Autodesk Inventor part; units mm, degrees
ref_plane "YZ Plane" through (0, 0, 0) normal (1, 0, 0) x (0, 1, 0)
ref_plane "XZ Plane" through (0, 0, 0) normal (0, 1, 0) x (-1, 0, 0)
ref_plane "XY Plane" through (0, 0, 0) normal (0, 0, 1) x (1, 0, 0)
sketch "Sketch1" plane through (0, 0, 0) normal (0, 1, 0) x (-1, 0, 0)
  line L0 (0, 0) -> (170, 0)
  line L1 (170, 0) -> (170, 10)
  line L2 (170, 10) -> (0, 10)
  line L3 (0, 10) -> (0, 0)
  dimension "d0" = 170
  dimension "d1" = 10
extrude "Extrusion1" add sketch "Sketch1" along normal blind 10
sketch "Sketch2" plane through (0, 10, 0) normal (0, 1, 0) x (1, 0, 0)
  line L0 (0, -10) -> (0, 0)
  line L1 (0, -5) -> (-2.2, -5)
  circle A0 centre (-6.1, -5) radius 3.9
  line L2 (0, 0) -> (-170, 0)
  line L3 (-170, -10) -> (0, -10)
  circle A1 centre (-75, -5) radius 1.5
  circle A2 centre (-95, -5) radius 1.5
  dimension "d4" = 2.2
  dimension "d8" = 3
  dimension "d9" = 3
extrude "Extrusion2" cut sketch "Sketch2" against normal blind 10 contours A1
extrude "Extrusion3" cut sketch "Sketch2" against normal blind 10 contours A2
extrude "Extrusion4" cut sketch "Sketch2" against normal blind 10 contours A0
sketch "Sketch3" plane through (0, 10, 0) normal (0, 1, 0) x (1, 0, 0)
  line L0 (-170, 0) -> (-170, -10)
  line L1 (-170, -5) -> (-10, -5)
  circle A0 centre (-6.1, -5) radius 3.9
  line L2 (-165.7, -5) -> (-163.45, -5)
  circle A1 centre (-163.45, -5) radius 2.25
  circle A2 centre (-153.45, -5) radius 2.25
  circle A3 centre (-143.45, -5) radius 2.25
  circle A4 centre (-133.45, -5) radius 2.25
  circle A5 centre (-123.45, -5) radius 2.25
  circle A6 centre (-113.45, -5) radius 2.25
  circle A7 centre (-103.45, -5) radius 2.25
  circle A8 centre (-95, -5) radius 1.5
  line L3 (-93.5, -5) -> (-93.5, -7.9104)
  circle A9 centre (-75, -5) radius 1.5
  line L4 (-76.5, -5) -> (-76.5, -7.25)
  line L5 (-93.5, -5) -> (-76.5, -5)
  line L6 (-85, -5) -> (-93.5, -5)
  line L7 (-85, -5) -> (-76.5, -5)
  circle A10 centre (-80.75, -5) radius 2.25
  circle A11 centre (-89.25, -5) radius 2.25
  line L8 (-10, -5) -> (-12, -5)
  line L9 (-10, -5) -> (-14.3, -5)
  line L10 (-14.3, -5) -> (-16.55, -5)
  circle A12 centre (-16.55, -5) radius 2.25
  circle A13 centre (-26.55, -5) radius 2.25
  circle A14 centre (-36.55, -5) radius 2.25
  circle A15 centre (-46.55, -5) radius 2.25
  circle A16 centre (-56.55, -5) radius 2.25
  circle A17 centre (-66.55, -5) radius 2.25
  point P0 (0, 0)
  point P1 (-155.7, -5)
  point P2 (-145.7, -5)
  point P3 (-135.7, -5)
  point P4 (-125.7, -5)
  point P5 (-115.7, -5)
  point P6 (-105.7, -5)
  point P7 (-24.3, -5)
  point P8 (-34.3, -5)
  point P9 (-44.3, -5)
  point P10 (-54.3, -5)
  point P11 (-64.3, -5)
  dimension "d20" = 10
  dimension "d32" = 10
extrude "Extrusion5" cut sketch "Sketch3" against normal blind 10 contours A1 L1 | L1 A1 | L1 A12 | L1 A12 | A2 L1 | L1 A2 | A3 L1 | L1 A3 | A4 L1 | L1 A4 | A5 L1 | L1 A5 | A6 L1 | L1 A6 | A7 L1 | L1 A7 | A11 L1 | L1 A11 | A10 L1 | L1 A10 | A17 L1 | L1 A17 | A16 L1 | L1 A16 | A15 L1 | L1 A15 | A14 L1 | L1 A14 | A13 L1 | L1 A13
thread "Thread1"
thread "Thread2"
sketch "Sketch4" plane through (0, 10, 0) normal (0, 1, 0) x (1, 0, 0)
  circle A0 centre (-16.55, -5) radius 2.25
  circle A1 centre (-16.55, -5) radius 2.25
  point P0 (0, 0)
extrude "Extrusion6" add sketch "Sketch4" against normal blind 10
sketch "Sketch5" plane through (0, 0, 10) normal (1, 0, 0) x (0, 0, -1)
  line L0 (10, 0) -> (0, 0)
  line L1 (0, 0) -> (0, 10)
  line L2 (10, 0) -> (0, 0)
  line L3 (0, 0) -> (0, 10)
  line L4 (0, 10) -> (10, 10)
  line L5 (10, 10) -> (10, 0)
extrude "Extrusion7" add sketch "Sketch5" along normal blind 10
sketch "Sketch6" plane through (10, 0, 10) normal (1, 0, 0) x (0, 0, -1)
  line L0 (0, 0) -> (10, 0)
  line L1 (0, 10) -> (0, 0)
  line L2 (10, 0) -> (0, 0)
  line L3 (0, 0) -> (0, 10)
  line L4 (0, 10) -> (10, 10)
  line L5 (10, 10) -> (10, 0)
extrude "Extrusion8" add sketch "Sketch6" along normal blind 10
sketch "Sketch7" plane through (0, 10, 0) normal (0, 1, 0) x (1, 0, 0)
  point P0 (0, 0)
fillet "Fillet3" radius 1 11 edges at (-75, 10, 10) (-75, 0, 10) (-75, 10, 0) (20, 5, 10) (20, 5, 0) (20, 0, 5) (-170, 10, 5) (-170, 5, 10) (-170, 5, 0) (-170, 0, 5) (-75, 0, 0)
fillet "Fillet4" radius 1 3 edges at (19.7071, 9.7071, 9.7071) (19.7071, 9.7071, 0.2929) (20, 10, 5)
sketch "Sketch8" plane through (19, 1, 0) normal (0, 0, -1) x (-1, 0, 0)
  point P0 (19, -1)
sketch "Sketch9" plane through (0, 10, 0) normal (0, 1, 0) x (1, 0, 0)
  circle A0 centre (-6.1, -5) radius 3.9
  circle A1 centre (-6.1, -5) radius 2.5
  point P0 (0, 0)
  dimension "d53" = 5
extrude "Extrusion9" add sketch "Sketch9" against normal blind 10
sketch "Sketch10" plane through (0, 10, 0) normal (0, 1, 0) x (1, 0, 0)
  circle A0 centre (-6.1, -5) radius 2.5
  line L0 (-3.6, -5) -> (1.4, -5)
  line L1 (19, -9) -> (19, -1)
  line L2 (1.4, -5) -> (-76.5, -5)
  circle A1 centre (-75, -5) radius 1.5
  line L3 (-76.5, -5) -> (-76.5, -10.0231)
  line L4 (-76.5, -10.0231) -> (-76.5, 0)
  line L5 (-76.5, -10.0231) -> (-169.9715, -10.0231)
  line L6 (-169, -9) -> (19, -9)
  line L7 (-169.9715, 0) -> (-76.5, 0)
  line L8 (-169.9715, -10.0231) -> (-170.1763, -9.372)
  line L9 (-170.1763, -9.372) -> (-170.4489, -3.7164)
  line L10 (-170.4489, -3.7164) -> (-170.4593, -3.5)
  line L11 (-170.4593, -3.5) -> (-170.4593, -0.543)
  line L12 (-170.4593, -0.543) -> (-169.9715, 0)
  point P0 (0, 0)
  dimension "d56" = 5
extrude "Extrusion10" cut sketch "Sketch10" against normal blind 10 contours L3 L5 L8 L9 L10 L11 L12 L7 L4
sketch "Sketch11" plane through (0, 10, 0) normal (0, 1, 0) x (1, 0, 0)
  circle A0 centre (-75, -5) radius 1.5
  circle A1 centre (-75, -5) radius 1.5
  circle A2 centre (-66.55, -5) radius 2.25
  circle A3 centre (-66.55, -5) radius 2.25
  circle A4 centre (-56.55, -5) radius 2.25
  circle A5 centre (-56.55, -5) radius 2.25
  circle A6 centre (-46.55, -5) radius 2.25
  circle A7 centre (-46.55, -5) radius 2.25
  circle A8 centre (-36.55, -5) radius 2.25
  circle A9 centre (-36.55, -5) radius 2.25
  circle A10 centre (-26.55, -5) radius 2.25
  circle A11 centre (-26.55, -5) radius 2.25
  point P0 (0, 0)
  point P1 (-76.5, -5)
extrude "Extrusion11" add sketch "Sketch11" against normal blind 10
sketch "Sketch12" plane through (0, 10, 0) normal (0, 1, 0) x (1, 0, 0)
  circle A0 centre (-6.1, -5) radius 2.5
  line L0 (-8.6, -5) -> (-76.5, -5)
  line L1 (-76.5, -9) -> (-76.5, -1)
  line L2 (-42.55, -5) -> (-27.55, -5)
  line L3 (-42.55, -5) -> (-57.55, -5)
  line L4 (-42.55, -5) -> (-50.05, -5)
  line L5 (-42.55, -5) -> (-35.05, -5)
  circle A1 centre (-50.05, -5) radius 1.5
  circle A2 centre (-35.05, -5) radius 1.5
  line L6 (-3.6, -5) -> (6.4143, -5)
  line L7 (6.4143, -5) -> (6.4143, -10.3738)
  line L8 (6.4143, -10.3738) -> (6.4143, 1.3096)
  line L9 (6.4143, 1.3096) -> (23.7189, 1.3096)
  line L10 (23.7189, 1.3096) -> (24.3802, -13.5702)
  line L11 (24.3802, -13.5702) -> (6.4143, -10.3738)
  point P0 (0, 0)
  dimension "d61" = 15
  dimension "d62" = 15
  dimension "d63" = 3
  dimension "d64" = 3
extrude "Extrusion12" cut sketch "Sketch12" against normal blind 10 contours A2 L0 | L0 A2 | A1 L0 | L0 A1 | L8 L9 L10 L11 L7
sketch "Sketch13" plane through (0, 10, 0) normal (0, 1, 0) x (1, 0, 0)
  circle A0 centre (-50.05, -5) radius 1.5
  line L0 (-48.55, -5) -> (-36.55, -5)
  circle A1 centre (-35.05, -5) radius 1.5
  circle A2 centre (-42.55, -5) radius 2.25
  line L1 (-51.55, -5) -> (-55.25, -5)
  line L2 (-33.55, -5) -> (-29.85, -5)
  circle A3 centre (-57.5, -5) radius 2.25
  circle A4 centre (-27.6, -5) radius 2.25
  circle A5 centre (-20.9, -5) radius 2.25
  circle A6 centre (-14.2, -5) radius 2.25
  circle A7 centre (-64.2, -5) radius 2.25
  circle A8 centre (-70.9, -5) radius 2.25
  point P0 (0, 0)
  dimension "d67" = 4.5
  dimension "d68" = 3.7
  dimension "d69" = 3.7
  dimension "d71" = 4.5
  dimension "d73" = 4.5
  dimension "d83" = 6.7
  dimension "d90" = 6.7
extrude "Extrusion13" cut sketch "Sketch13" against normal blind 10 contours A3 | A4 | A5 | A6 | A7 | A8
sketch "Sketch14" plane through (0, 10, 0) normal (0, 1, 0) x (1, 0, 0)
  circle A0 centre (-57.5, -5) radius 2.25
  line L0 (-55.25, -5) -> (-29.85, -5)
  circle A1 centre (-27.6, -5) radius 2.25
  circle A2 centre (-42.55, -5) radius 2.25
  point P0 (0, 0)
  dimension "d97" = 4.5
extrude "Extrusion14" cut sketch "Sketch14" against normal blind 10 contours A2 L0 | L0 A2
thread "Thread3"
thread "Thread4"
fillet "Fillet5" radius 1 16 edges at (-76.5, 9.7071, 9.7071) (-76.5, 5, 10) (-76.5, 0.2929, 9.7071) (-76.5, 0, 5) (-76.5, 0.2929, 0.2929) (-76.5, 5, 0) (-76.5, 9.7071, 0.2929) (-76.5, 10, 5) (6.4143, 9.7071, 0.2929) (6.4143, 5, 0) (6.4143, 0.2929, 0.2929) (6.4143, 0, 5) (6.4143, 0.2929, 9.7071) (6.4143, 5, 10) (6.4143, 9.7071, 9.7071) (6.4143, 10, 5)
sketch "Sketch15" plane through (0, 10, 0) normal (0, 1, 0) x (1, 0, 0)
  circle A0 centre (-6.1, -5) radius 2.5
  circle A1 centre (-6.1, -5) radius 2.75
  point P0 (0, 0)
  dimension "d105" = 5.5
extrude "Extrusion15" cut sketch "Sketch15" against normal blind 10 contours A0 | A1
properties part number "brazo de servo el d vdd - camara"
Part model, mm, in its own coordinate system. Round coordinates to 2 decimals unless told otherwise and drop trailing zeros. Loops run counter-clockwise (first coordinate to the right, second up) from the corner with the lowest first, then second, coordinate; pieces in that order, holes last. Notation, with made-up numbers: (26.25, 67) -> (38.25, 67) arc R17 ccw to (38.25, 87) -> close; hole circle Ø1 at (-30.5, 75). An arc over 180 degrees is marked (long way). Use one line per item in the form item = value. Start each with the question number.
Item 1: Band-saw the part on A-A (x = -42.55). List the corners of the cut face in (y, z).
Item 2: Band-saw the part on C-C (x = -29). List the corners of the cut face in (y, z).
Item 3: Drop a flat-ended pin along its axis: pin 1 Ø3.5 at (x, z) = (-57.5, 5) entering from -Y. Give the stop position or say it passes through.
Item 4: Two-plate mould, pull along Z, no slides. Class faces 1 (the flat face through (-36, 5, 0)), 2 (the flat face through (-36, 5, 10)), 3 (the cylindrical face through (-51.24, 5.07, 5.91)), 4 (the flat face through (-36, 0, 7)): released by +Z, released by -Z, zero draft, split by the parting line, or undercut.
Item 5: Drill centre lines: line 1 along Z through (x, y) = (-50.05, 2.25); line 2 along Z through (x, y) = (-14.2, 7.75); line 3 along X through (y, z) = (1.25, 9.25). Where is each one in solid material? Low to high.
Item 6: Band-saw the part on B-B (y = 4). Give the number of separate pieces and of enclosed holes in the cut face, plus the area to 3 significant figures.
Data:
q1.outline = (0, 1) arc R1 ccw to (1, 0) -> (9, 0) arc R1 ccw to (10, 1) -> (10, 2.75) -> (0, 2.75) -> close; (0, 7.25) -> (10, 7.25) -> (10, 9) arc R1 ccw to (9, 10) -> (1, 10) arc R1 ccw to (0, 9) -> close
q2.outline = (0, 1) arc R1 ccw to (1, 0) -> (9, 0) arc R1 ccw to (10, 1) -> (10, 3.24) -> (0, 3.24) -> close; (0, 6.76) -> (10, 6.76) -> (10, 9) arc R1 ccw to (9, 10) -> (1, 10) arc R1 ccw to (0, 9) -> close
q3.pin_1 = through
q4.face_1 = released by -Z
q4.face_2 = released by +Z
q4.face_3 = undercut
q4.face_4 = zero draft
q5.line_1 = 0 to 3.5, 6.5 to 10
q5.line_2 = 0 to 2.75, 7.25 to 10
q5.line_3 = -76.47 to 6.38
q6.separate_pieces = 1
q6.enclosed_holes = 10
q6.area = 679 mm^2
